from build123d import *

# Parameters (mm, degrees)
ESQUISSE1_W             = 430
ESQUISSE1_H             = 10
BOSS_EXTRU_1_DEPTH      = 5
ENL_V_MAT_EXTRU_1_REACH = 7


with BuildPart() as part:
    # Esquisse1 → Boss.-Extru.1 (new body)
    with BuildSketch(Plane.XY):
        Polygon((0, 50), (5, 50), (5, 0), (495, 0), (495, 50), (500, 50), (500, 100), (495, 100), (495, 150), (500, 150), (500, 183), (0, 183), (0, 150), (5, 150), (5, 100), (0, 100), align=None)
        with Locations((250, 110)):
            Rectangle(ESQUISSE1_W, ESQUISSE1_H, mode=Mode.SUBTRACT)
    extrude(amount=BOSS_EXTRU_1_DEPTH)

    # Esquisse2 → Enlèv. mat.-Extru.1 (cut, up to next)
    with BuildSketch(Plane(origin=(0, 0, 0), x_dir=(-1, 0, 0), z_dir=(0, 0, -1)), mode=Mode.PRIVATE) as enl_v_mat_extru_1_sk1:
        with BuildLine():
            Line((-483, 30), (-477, 30))
            ThreePointArc((-477, 30), (-475.585786438, 30.585786438), (-475, 32))
            Line((-475, 32), (-475, 48))
            ThreePointArc((-475, 48), (-475.585786438, 49.414213562), (-477, 50))
            Line((-477, 50), (-483, 50))
            ThreePointArc((-483, 50), (-484.414213562, 49.414213562), (-485, 48))
            Line((-485, 48), (-485, 32))
            ThreePointArc((-485, 32), (-484.414213562, 30.585786438), (-483, 30))
        make_face()
    enl_v_mat_extru_1_tool1 = extrude(enl_v_mat_extru_1_sk1.sketch, amount=-ENL_V_MAT_EXTRU_1_REACH, mode=Mode.PRIVATE) & part.part
    add(enl_v_mat_extru_1_tool1.solids().sort_by_distance((480, 40, 0))[0], mode=Mode.SUBTRACT)


solid = part.part
Here's how the part is built. I have some questions about the finished solid (model axes, mm). Round coordinates to 2 decimals unless told otherwise and drop trailing zeros. Loops run counter-clockwise (first coordinate to the right, second up) from the corner with the lowest first, then second, coordinate; pieces in that order, holes last. Notation, with made-up numbers: (47, -27) -> (98, -27) arc R19 ccw to (98, -21) -> close; hole circle Ø2 at (-8.75, -31). An arc over 180 degrees is marked (long way). Write each question's results on one line, items separated by ' | '.
(1) If we section it at A-A, the plane z = 3.9: List the corners of the cut face in (x, y) for me, then the cut area to 3 significant figures.
Worked answers:
outline: (0, 50) -> (5, 50) -> (5, 0) -> (495, 0) -> (495, 50) -> (500, 50) -> (500, 100) -> (495, 100) -> (495, 150) -> (500, 150) -> (500, 183) -> (0, 183) -> (0, 150) -> (5, 150) -> (5, 100) -> (0, 100) -> close; hole (35, 105) -> (465, 105) -> (465, 115) -> (35, 115) -> close; hole (475, 32) arc R2 ccw to (477, 30) -> (483, 30) arc R2 ccw to (485, 32) -> (485, 48) arc R2 ccw to (483, 50) -> (477, 50) arc R2 ccw to (475, 48) -> close | area: 86,000 mm2
(2) If we section it at B-B, the plane x = 341: List the corners of the cut face in (y, z) for me, then the cut area to 3 significant figures.
Worked answers:
outline: (0, 0) -> (105, 0) -> (105, 5) -> (0, 5) -> close; (115, 0) -> (183, 0) -> (183, 5) -> (115, 5) -> close | area: 865 mm2
(3) For P1, Ø1, axis at y = 127, z = 1.5, coming from the -X side; P2, Ø2.5, axis at x = 498, z = 2, coming from the -Y side; P3, Ø3, axis at x = 75, z = 0.5, coming from the -Y side; P4, Ø2.5, axis at y = 42, z = 3, coming from the +X side, each with a flat end and sliding along its axis, tell me the tip position at first contact or that it passes through.
Worked answers:
P1: x = 5 | P2: y = 50 | P3: y = 0 | P4: x = 495
(4) If I drill on L1, parallel to Y at x = 138.5, z = 2.7; L2, parallel to X at y = 109, z = 1.6; L3, parallel to X at y = 124, z = 3.8, over which ranges is the centre line in solid material (lowest first)?
Worked answers:
L1: 0 to 105, 115 to 183 | L2: 5 to 35, 465 to 495 | L3: 5 to 495
(5) If we section it at C-C, the plane y = 142: List the corners of the cut face in (x, z) for me, then the cut area to 3 significant figures.
Worked answers:
outline: (5, 0) -> (495, 0) -> (495, 5) -> (5, 5) -> close | area: 2,450 mm2
